```python
from build123d import *

# Parameters (mm, degrees)
EXTRUDE_1_DEPTH     = 10.6
SKETCH_2_R          = 1
CUT_EXTRUDE_1_DEPTH = 14.637927158


with BuildPart() as part:
    # 草图1 → 凸台-拉伸1 (new body)
    with BuildSketch(Plane.XY):
        Polygon((-8.25, 0), (8.25, 0), (8.25, 2), (0, 2.360202779), (-8.25, 2), align=None)
    extrude(amount=EXTRUDE_1_DEPTH)

    # 草图2 → 切除-拉伸1 (cut, through all)
    with BuildSketch(Plane.XZ):
        with Locations((4, 5.3)):
            Circle(SKETCH_2_R)
        with Locations(Location((-4, 5.3, 0), (0, 0, 180))):
            Circle(SKETCH_2_R)
    extrude(amount=-CUT_EXTRUDE_1_DEPTH, mode=Mode.SUBTRACT)


solid = part.part
```
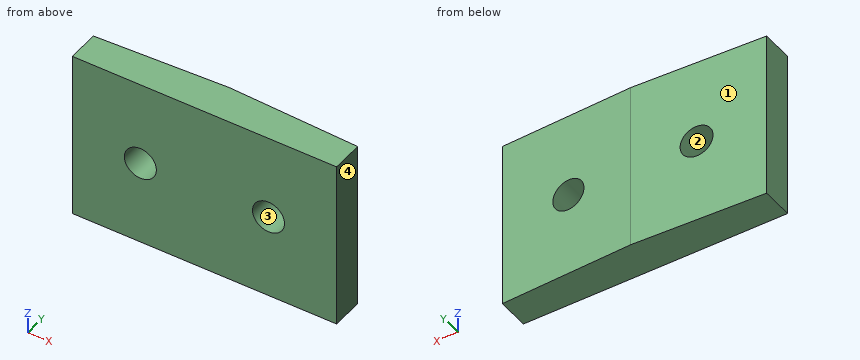
For this review, take the finished solid that the model builds, in its own axes (mm). Face numbers are marked on the shaded views. Give positions to 0.01 mm unless a question says otherwise; leave off trailing zeros. Loops run counter-clockwise (first coordinate to the right, second up) from the corner with the lowest first, then second, coordinate; pieces in that order, holes last. Notation, with made-up numbers: M 89.5,-40 L 141.5,-40 A12 ccw 141.5,-29 Z; hole C 68.5,43 d3. An arc over 180 degrees is marked long. One line per item, written item: value. Start each with the question number.
Q1. Clearance check with a flat-ended pin moving along its axis: pin 1 Ø3 at (x, z) = (-4, 5.3) entering from +Y. State where the tip first meets the part, or that it passes through.
Q2. Add section D-D (x = -3.25). Give the boundary of the cut face in (y, z), and give its area (3 significant figures).
Q3. Add section A-A (x = 4). Give the boundary of the cut face in (y, z), and give its area (3 significant figures).
Q4. Add section C-C (y = 0.75). Give the boundary of the cut face in (x, z), and give its area (3 significant figures).
Q5. Add section B-B (z = 5.5). Give the boundary of the cut face in (x, y), and give its area (3 significant figures).
Q6. For L1, parallel to X at y = 1.3, z = 5.3; L2, parallel to Z at x = -4, y = 0.9; L3, parallel to X at y = 0.7, z = 6, list the stretches that pass through material, from the lowest coordinate up.
Q7. Draft analysis for pull direction X (two halves, no side actions). For the marked faces 1, 2, 3 and 4, state which applies: released by +X, released by -X, zero draft, split by the parting line, or undercut.
Reply:
1. pin 1: y = 2.25
2. outline: M 0,0 L 2.22,0 L 2.22,4.64 L 0,4.64 Z; M 0,5.96 L 2.22,5.96 L 2.22,10.6 L 0,10.6 Z
2. area: 20.6 mm²
3. outline: M 0,0 L 2.19,0 L 2.19,4.3 L 0,4.3 Z; M 0,6.3 L 2.19,6.3 L 2.19,10.6 L 0,10.6 Z
3. area: 18.8 mm²
4. outline: M -8.25,0 L 8.25,0 L 8.25,10.6 L -8.25,10.6 Z; hole C -4,5.3 d2; hole C 4,5.3 d2
4. area: 169 mm²
5. outline: M -8.25,0 L -4.98,0 L -4.98,2.14 L -8.25,2 Z; M -3.02,0 L 3.02,0 L 3.02,2.23 L 0,2.36 L -3.02,2.23 Z; M 4.98,0 L 8.25,0 L 8.25,2 L 4.98,2.14 Z
5. area: 27.4 mm²
6. L1: -8.25 to -5, -3 to 3, 5 to 8.25
6. L2: 0 to 4.3, 6.3 to 10.6
6. L3: -8.25 to -4.71, -3.29 to 3.29, 4.71 to 8.25
7. face 1: released by -X
7. face 2: undercut
7. face 3: undercut
7. face 4: released by +X
